```python
from build123d import *

# Parameters (mm, degrees)
FLEXURE_BOSS_DEPTH            = 5
SKETCH2_W                     = 10.32
SKETCH2_H                     = 18
SKETCH2_R                     = 1.575
MOUNTING_PLATE_BOSS_DEPTH     = 1.5
DOVETAIL_CONNECTION_CUT_DEPTH = 3.455


with BuildPart() as part:
    # Sketch1 → Flexure Boss (new body)
    with BuildSketch(Plane(origin=(0, 0, 0), x_dir=(0, 0, -1), z_dir=(1, 0, 0))):
        with BuildLine():
            Line((3.743651747, -1.066915143), (8.368651984, -1.066915143))
            Line((8.368651984, -1.066915143), (8.368651984, 5.083084857))
            Line((8.368651984, 5.083084857), (-4.631348016, 5.083084857))
            Line((-4.631348016, 5.083084857), (-4.631348016, -1.066915143))
            Line((-4.631348016, -1.066915143), (-1.881348253, -1.066915143))
            ThreePointArc((-1.881348253, -1.066915143), (-1.174241471, -1.359808362), (-0.881348253, -2.066915143))
            Line((-0.881348253, -2.066915143), (-0.881348253, -10.941915143))
            Line((-0.881348253, -10.941915143), (3.368651984, -10.941915143))
            Line((3.368651984, -10.941915143), (3.368651984, -11.691915143))
            Line((3.368651984, -11.691915143), (-0.631348016, -11.691915143))
            ThreePointArc((-0.631348016, -11.691915143), (-1.338454797, -11.399021924), (-1.631348016, -10.691915143))
            Line((-1.631348016, -10.691915143), (-1.631348016, -1.566915143))
            Line((-1.631348016, -1.566915143), (-3.631348016, -1.566915143))
            Line((-3.631348016, -1.566915143), (-3.631348016, -11.816915143))
            ThreePointArc((-3.631348016, -11.816915143), (-4.070687844, -12.877575315), (-5.131348016, -13.316915143))
            Line((-5.131348016, -13.316915143), (-6.391348016, -13.316915143))
            Line((-6.391348016, -13.316915143), (-6.391348016, -19.646915143))
            Line((-6.391348016, -19.646915143), (-1.391348016, -19.646915143))
            Line((-1.391348016, -19.646915143), (-1.391348016, -18.146915143))
            Line((-1.391348016, -18.146915143), (-4.891348016, -18.146915143))
            Line((-4.891348016, -18.146915143), (-4.891348016, -14.816915143))
            Line((-4.891348016, -14.816915143), (-4.631348016, -14.816915143))
            Line((-4.631348016, -14.816915143), (14.675469929, -14.816915143))
            Line((14.675469929, -14.816915143), (14.675469929, -13.316915143))
            Line((14.675469929, -13.316915143), (13.993651747, -1.316915143))
            Line((13.993651747, -1.316915143), (11.993651747, -1.316915143))
            Line((11.993651747, -1.316915143), (11.993651747, -11.816915143))
            Line((11.993651747, -11.816915143), (11.743651747, -11.816915143))
            ThreePointArc((11.743651747, -11.816915143), (11.390098357, -11.670468534), (11.243651747, -11.316915143))
            Line((11.243651747, -11.316915143), (11.243651747, -1.816915143))
            Line((11.243651747, -1.816915143), (8.743651747, -1.816915143))
            Line((8.743651747, -1.816915143), (8.743651747, -2.316915143))
            Line((8.743651747, -2.316915143), (3.243651747, -2.316915143))
            Line((3.243651747, -2.316915143), (3.243651747, -4.316915143))
            Line((3.243651747, -4.316915143), (8.743651747, -4.316915143))
            Line((8.743651747, -4.316915143), (8.743651747, -4.816915143))
            ThreePointArc((8.743651747, -4.816915143), (8.670428443, -4.993691838), (8.493651747, -5.066915143))
            Line((8.493651747, -5.066915143), (2.743651747, -5.066915143))
            Line((2.743651747, -5.066915143), (2.743651747, -2.066915143))
            ThreePointArc((2.743651747, -2.066915143), (3.036544966, -1.359808362), (3.743651747, -1.066915143))
        make_face()
        with BuildLine():
            Line((0.243651747, -9.566915143), (9.868651747, -9.566915143))
            Line((9.868651747, -9.566915143), (9.868651747, -3.691915143))
            Line((9.868651747, -3.691915143), (4.243651747, -3.691915143))
            Line((4.243651747, -3.691915143), (4.243651747, -2.941915143))
            Line((4.243651747, -2.941915143), (9.618651747, -2.941915143))
            ThreePointArc((9.618651747, -2.941915143), (10.325758529, -3.234808362), (10.618651747, -3.941915143))
            Line((10.618651747, -3.941915143), (10.618651747, -12.816915143))
            Line((10.618651747, -12.816915143), (12.618651747, -12.816915143))
            Line((12.618651747, -12.816915143), (12.618651747, -2.316915143))
            Line((12.618651747, -2.316915143), (13.368651747, -2.316915143))
            Line((13.368651747, -2.316915143), (13.948620781, -12.524370125))
            ThreePointArc((13.948620781, -12.524370125), (13.744993017, -13.0819837), (13.199828472, -13.316915143))
            Line((13.199828472, -13.316915143), (-1.506348016, -13.316915143))
            ThreePointArc((-1.506348016, -13.316915143), (-2.567008187, -12.877575315), (-3.006348016, -11.816915143))
            Line((-3.006348016, -11.816915143), (-3.006348016, -2.566915143))
            Line((-3.006348016, -2.566915143), (-2.256348016, -2.566915143))
            Line((-2.256348016, -2.566915143), (-2.256348016, -12.816915143))
            Line((-2.256348016, -12.816915143), (0.243651984, -12.816915143))
            Line((0.243651984, -12.816915143), (0.243651984, -12.316915143))
            Line((0.243651984, -12.316915143), (4.368651984, -12.316915143))
            Line((4.368651984, -12.316915143), (4.368651984, -10.316915143))
            Line((4.368651984, -10.316915143), (-0.006348253, -10.316915143))
            Line((-0.006348253, -10.316915143), (-0.006348253, -9.816915143))
            ThreePointArc((-0.006348253, -9.816915143), (0.066875052, -9.640138448), (0.243651747, -9.566915143))
        make_face(mode=Mode.SUBTRACT)
    extrude(amount=FLEXURE_BOSS_DEPTH)

    # Sketch2 → Mounting Plate Boss (add)
    with BuildSketch(Plane.XZ.offset(14.816915143)):
        with Locations((-0.16, -16.309568548)):
            Rectangle(SKETCH2_W, SKETCH2_H)
        with Locations(Location((-2.435, -10.088651984, 0), (0, 0, 270))):
            Circle(SKETCH2_R, mode=Mode.SUBTRACT)
        with Locations(Location((-2.435, -22.088651984, 0), (0, 0, 270))):
            Circle(SKETCH2_R, mode=Mode.SUBTRACT)
    extrude(amount=-MOUNTING_PLATE_BOSS_DEPTH)

    # Sketch7 → Dovetail Connection Cut (cut)
    with BuildSketch(Plane.ZY):
        Polygon((-8.368651984, 0.933084857), (4.631348016, 0.933084857), (4.631348016, 4.083084857), (-1.868651984, 3.083084857), (-8.368651984, 4.083084857), align=None)
    extrude(amount=-DOVETAIL_CONNECTION_CUT_DEPTH, mode=Mode.SUBTRACT)


solid = part.part
```
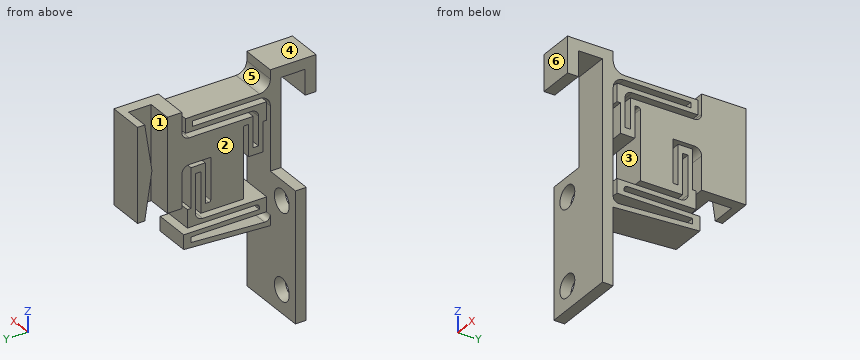
Source: CAD feature listing. Evaluate the final solid. Frame: model axes, mm. Face numbers are marked on the shaded views. A direction names the side the tool comes from. Round coordinates to 2 decimals unless told otherwise and drop trailing zeros. Loops run counter-clockwise (first coordinate to the right, second up) from the corner with the lowest first, then second, coordinate; pieces in that order, holes last.
(1) Section query D-D (y = -8). Output: boundary loops of the cut face in (x, z), and give its area (3 significant figures).
From the geometry:
outline: (0, -14.37) - (5, -14.37) - (5, -13.69) - (0, -13.69) - close; (0, -12.62) - (5, -12.62) - (5, -11.99) - (0, -11.99) - close; (0, -11.24) - (5, -11.24) - (5, -10.62) - (0, -10.62) - close; (0, -9.87) - (5, -9.87) - (5, 0.88) - (0, 0.88) - close; (0, 1.63) - (5, 1.63) - (5, 2.26) - (0, 2.26) - close; (0, 3.01) - (5, 3.01) - (5, 3.63) - (0, 3.63) - close
area: 69.7 mm2
(2) Section query C-C (z = -21.5). Output: boundary loops of the cut face in (x, y), and give its area (3 significant figures).
From the geometry:
outline: (-5.32, -14.82) - (-3.9, -14.82) - (-3.9, -13.32) - (-5.32, -13.32) - close; (-0.97, -14.82) - (5, -14.82) - (5, -13.32) - (-0.97, -13.32) - close
area: 11.1 mm2
(3) Access query for the marked faces 1, 2 and 3. Directions: +Z, -Z, +X, -X, +Y, -Y. A direction counts if a zero-diameter tool reaches every point of the face in a straight line with its end or side. Return the directions, or none.
From the geometry:
face 1: +Z, -Z, -X
face 2: +Z, -X, +Y
face 3: +X, -X
(4) Section query A-A (z = 4). Output: boundary loops of the cut face in (x, y) (3 decimals).
From the geometry:
outline: (0, -19.647) - (5, -19.647) - (5, -18.147) - (0, -18.147) - close; (0, -14.817) - (5, -14.817) - (5, -12.802) - (0, -12.802) - close; (0, -1.067) - (5, -1.067) - (5, 5.083) - (0, 5.083) - (0, 3.986) - (3.455, 3.986) - (3.455, 0.933) - (0, 0.933) - close
(5) Contact query for flat-ended pins moving along their axis: pin 1 Ø1.5 at (x, z) = (-0.5, -18) entering from +Y; pin 2 Ø1.2 at (x, z) = (2, -9.5) entering from +Y; pin 3 Ø0.6 at (y, z) = (4, -4) entering from -X. Output: stop coordinate, or through.
From the geometry:
pin 1: stops at y = -13.32
pin 2: stops at y = -1.82
pin 3: stops at x = 0
(6) Section query B-B (x = 0.5). Give the number of separate pieces and of enclosed holes in the cut face, and give its area (3 significant figures).
From the geometry:
separate pieces: 2
enclosed holes: 1
area: 230 mm2
(7) Pull-direction query (Y, two-part tool) for the marked faces 4, 5 and 6; classes: +Y half, -Y half, draft (parallel to the pull), parting line (faces both ways), or undercut.
From the geometry:
face 4: draft
face 5: undercut
face 6: -Y half
(8) Material intervals for probe 1 along Z at (x, y) = (-2.75, -14.25); probe 2 along Y at (x, z) = (0.75, -5); probe 3 along Y at (x, z) = (0.75, -15.5), sorted ascending.
From the geometry:
probe 1: z = -25.31 to -23.63, -20.55 to -11.63, -8.55 to -7.31
probe 2: y = -14.82 to -13.32, -9.57 to -5.07, -4.32 to -3.69, -2.94 to -2.32, -1.07 to 0.93, 3.56 to 5.08
probe 3: y = -14.82 to -13.32
